Geometry: see drawing. Coordinates: mm, zero at the bounding-box minimum. Give positions to 0.01 mm unless a question says otherwise; leave off trailing zeros. Write each loop counter-clockwise with the first axis right and the second up, starting at its lowest first coordinate (ties: lowest second). Pieces come first, ordered by that corner, then holes.
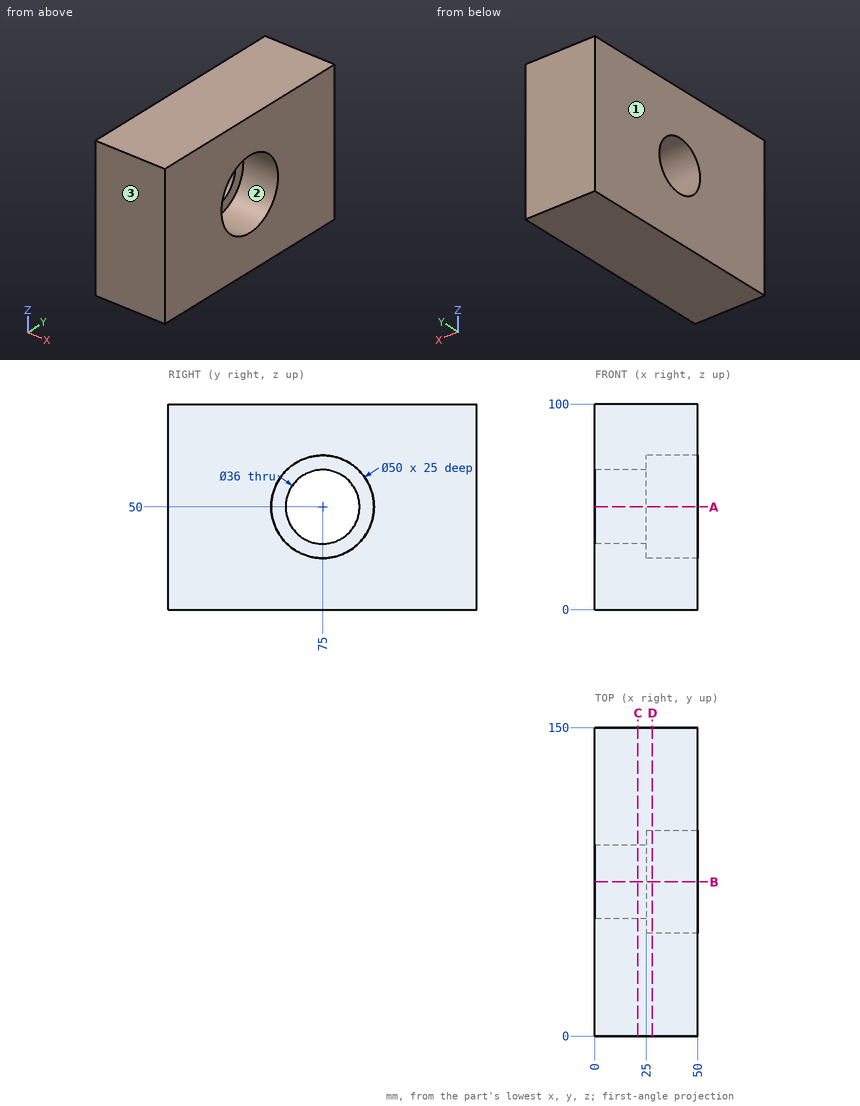
Q1. Section D-D, the plane x = 28. Return the cut outline in (y, z).
Q2. Section C-C, the plane x = 21. Return the cut outline in (y, z), then the cut area to 3 significant figures.
Q3. Section A-A, the plane z = 50. Return the cut outline in (x, y).
Q4. Section B-B, the plane y = 75. Return the cut outline in (x, z), then the cut area to 3 significant figures.
Q5. Mould query, pull axis Y, two halves, no side actions, for the marked faces 1, 2 and 3. Classes: +Y half, -Y half, draft (parallel to the pull), parting line (faces both ways), or undercut.
Q6. Pin query (flat end, axial travel): pin 1 (25 mm diameter, centred on y = 82.5, z = 42, fed in from +X). Return the tip coordinate at first contact, or that it passes through.
Q7. Material intervals for line 1 along Z through (x, y) = (32, 75); line 2 along Y through (x, z) = (30, 50); line 3 along X through (y, z) = (97.5, 44), sorted ascending.
Solutions:
1. outline: (0, 0) - (150, 0) - (150, 100) - (0, 100) - close; hole circle Ø50 at (75, 50)
2. outline: (0, 0) - (150, 0) - (150, 100) - (0, 100) - close; hole circle Ø36 at (75, 50)
2. area: 14,000 mm2
3. outline: (0, 0) - (50, 0) - (50, 50) - (25, 50) - (25, 57) - (0, 57) - close; (0, 93) - (25, 93) - (25, 100) - (50, 100) - (50, 150) - (0, 150) - close
4. outline: (0, 0) - (50, 0) - (50, 25) - (25, 25) - (25, 32) - (0, 32) - close; (0, 68) - (25, 68) - (25, 75) - (50, 75) - (50, 100) - (0, 100) - close
4. area: 2,850 mm2
5. face 1: draft
5. face 2: undercut
5. face 3: -Y half
6. pin 1: stops at x = 25
7. line 1: z = 0 to 25, 75 to 100
7. line 2: y = 0 to 50, 100 to 150
7. line 3: x = 0 to 25
